```python
from build123d import *

# Parameters (mm, degrees)
PAD026_DEPTH      = 130
CYLINDER004_R     = 2.7
CYLINDER004_DEPTH = 30
CYLINDER005_R     = 2.7
CYLINDER005_DEPTH = 30
CYLINDER006_R     = 2.7
CYLINDER006_DEPTH = 30
CYLINDER007_R     = 2.7
CYLINDER007_DEPTH = 30
CYLINDER008_R     = 2.7
CYLINDER008_DEPTH = 30
CYLINDER009_R     = 2.7
CYLINDER009_DEPTH = 30
CYLINDER010_R     = 3.2
CYLINDER010_DEPTH = 50
CYLINDER011_R     = 3.2
CYLINDER011_DEPTH = 40
CYLINDER012_R     = 3.2
CYLINDER012_DEPTH = 40
CYLINDER013_R     = 7.5
CYLINDER013_DEPTH = 13
CYLINDER014_R     = 7.5
CYLINDER014_DEPTH = 13
CYLINDER015_R     = 7.5
CYLINDER015_DEPTH = 13
FILLET021_R       = 3


with BuildPart() as part:
    # Sketch051 → Pad026 (new body)
    with BuildSketch(Plane.XZ):
        Polygon((0, 0), (0, 20), (20, 20), (68.296291, 7.059048), (71.763809, 20), (110, 20), (110, 0), align=None)
    extrude(amount=PAD026_DEPTH)

    # Cylinder004 → Cylinder004 (cut)
    with BuildSketch(Plane(origin=(9, -10, 0), x_dir=(1, 0, 0), z_dir=(0, 0, 1))):
        Circle(CYLINDER004_R)
    extrude(amount=CYLINDER004_DEPTH, mode=Mode.SUBTRACT)

    # Cylinder005 → Cylinder005 (cut)
    with BuildSketch(Plane(origin=(95, -20, 0), x_dir=(1, 0, 0), z_dir=(0, 0, 1))):
        Circle(CYLINDER005_R)
    extrude(amount=CYLINDER005_DEPTH, mode=Mode.SUBTRACT)

    # Cylinder006 → Cylinder006 (cut)
    with BuildSketch(Plane(origin=(95, -65, 0), x_dir=(1, 0, 0), z_dir=(0, 0, 1))):
        Circle(CYLINDER006_R)
    extrude(amount=CYLINDER006_DEPTH, mode=Mode.SUBTRACT)

    # Cylinder007 → Cylinder007 (cut)
    with BuildSketch(Plane(origin=(95, -110, 0), x_dir=(1, 0, 0), z_dir=(0, 0, 1))):
        Circle(CYLINDER007_R)
    extrude(amount=CYLINDER007_DEPTH, mode=Mode.SUBTRACT)

    # Cylinder008 → Cylinder008 (cut)
    with BuildSketch(Plane(origin=(9, -65, 0), x_dir=(1, 0, 0), z_dir=(0, 0, 1))):
        Circle(CYLINDER008_R)
    extrude(amount=CYLINDER008_DEPTH, mode=Mode.SUBTRACT)

    # Cylinder009 → Cylinder009 (cut)
    with BuildSketch(Plane(origin=(9, -120, 0), x_dir=(1, 0, 0), z_dir=(0, 0, 1))):
        Circle(CYLINDER009_R)
    extrude(amount=CYLINDER009_DEPTH, mode=Mode.SUBTRACT)

    # Cylinder010 → Cylinder010 (cut)
    with BuildSketch(Plane(origin=(38, -35, -5), x_dir=(0.965926, 0, -0.258819), z_dir=(0.258819, 0, 0.965926))):
        Circle(CYLINDER010_R)
    extrude(amount=CYLINDER010_DEPTH, mode=Mode.SUBTRACT)

    # Cylinder011 → Cylinder011 (cut)
    with BuildSketch(Plane(origin=(38, -65, -5), x_dir=(0.965926, 0, -0.258819), z_dir=(0.258819, 0, 0.965926))):
        Circle(CYLINDER011_R)
    extrude(amount=CYLINDER011_DEPTH, mode=Mode.SUBTRACT)

    # Cylinder012 → Cylinder012 (cut)
    with BuildSketch(Plane(origin=(38, -100, -5), x_dir=(0.965926, 0, -0.258819), z_dir=(0.258819, 0, 0.965926))):
        Circle(CYLINDER012_R)
    extrude(amount=CYLINDER012_DEPTH, mode=Mode.SUBTRACT)

    # Cylinder013 → Cylinder013 (cut)
    with BuildSketch(Plane(origin=(38, -35, -5), x_dir=(0.965926, 0, -0.258819), z_dir=(0.258819, 0, 0.965926))):
        Circle(CYLINDER013_R)
    extrude(amount=CYLINDER013_DEPTH, mode=Mode.SUBTRACT)

    # Cylinder014 → Cylinder014 (cut)
    with BuildSketch(Plane(origin=(38, -65, -5), x_dir=(0.965926, 0, -0.258819), z_dir=(0.258819, 0, 0.965926))):
        Circle(CYLINDER014_R)
    extrude(amount=CYLINDER014_DEPTH, mode=Mode.SUBTRACT)

    # Cylinder015 → Cylinder015 (cut)
    with BuildSketch(Plane(origin=(38, -100, -5), x_dir=(0.965926, 0, -0.258819), z_dir=(0.258819, 0, 0.965926))):
        Circle(CYLINDER015_R)
    extrude(amount=CYLINDER015_DEPTH, mode=Mode.SUBTRACT)

    # Fillet021
    fillet021_edges = [part.edges().sort_by_distance(p)[0] for p in [
        (0, -65, 20),
        (110, -65, 20),
        (0, -130, 10),
        (110, -130, 10),
        (0, 0, 10),
        (110, 0, 10),
        (90.881905, -130, 20),
        (90.881905, 0, 20),
        (10, -130, 20),
        (10, 0, 20),
    ]]
    fillet(fillet021_edges, radius=FILLET021_R)


solid = part.part
```
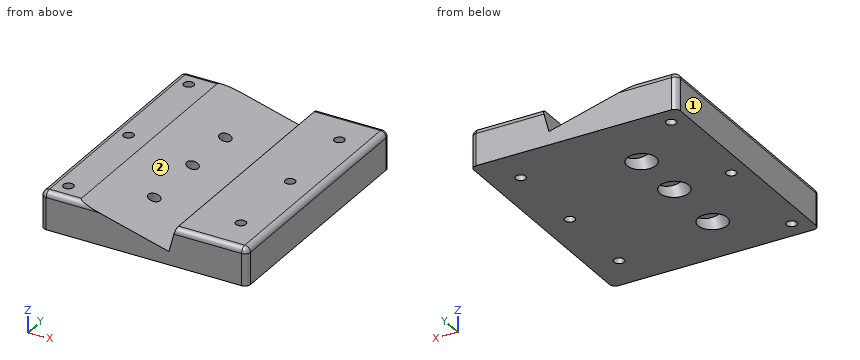
Part model, mm, in its own coordinate system. Face numbers are marked on the shaded views. A direction names the side the tool comes from. Coordinates: 2 decimals unless noted, no trailing zeros. Write each loop counter-clockwise with the first axis right and the second up, starting at its lowest first coordinate (ties: lowest second). Pieces come first, ordered by that corner, then holes.
Item 1: Which spindle directions (+Z, -Z, +X, -X, +Y, -Y) get a long thin tool onto all of the face, cutting with end or side? Do the marked faces 1 and 2. Say none if no direction does.
Item 2: Slice it at C-C (y = -65). Write the cut outline in (x, z).
Item 3: Slice it at D-D (y = -50). Write the cut outline in (x, z).
Item 4: Pin check, flat tip, straight feed: pin 1 (10 mm diameter, centred on x = 45, y = -32.5, fed in from +Z). Stop position of the tip, or through.
Item 5: Slice it at B-B (x = 95). Write the cut outline in (y, z), and give its area (3 significant figures).
Item 6: Slice it at A-A (y = -10). Write the cut outline in (x, z), and give its area (3 significant figures).
Item 7: Probe line 1 (Y direction, x = 9, z = 12); line 2 (Y direction, x = 95, z = 11.5); line 3 (X direction, y = -110, z = 6). List the from-to ranges inside material, lowest first.
Results found:
1. face 1: +Z, -Z, -X, +Y, -Y
1. face 2: +Z, +Y, -Y
2. outline: (0, 0) - (6.3, 0) - (6.3, 20) - (3, 20) arc R3 ccw to (0, 17) - close; (11.7, 0) - (31.58, 0) - (34.12, 9.5) - (38.27, 8.39) - (39.95, 14.65) - (20, 20) - (11.7, 20) - close; (44.46, 6.73) - (48.61, 5.62) - (47.1, 0) - (92.3, 0) - (92.3, 20) - (71.76, 20) - (68.3, 7.06) - (46.14, 13) - close; (97.7, 0) - (110, 0) - (110, 17) arc R3 ccw to (107, 20) - (97.7, 20) - close
3. outline: (0, 0) - (110, 0) - (110, 17) arc R3 ccw to (107, 20) - (71.76, 20) - (68.3, 7.06) - (20, 20) - (3, 20) arc R3 ccw to (0, 17) - close
4. pin 1: stops at z = 14.64
5. outline: (-130, 0) - (-112.7, 0) - (-112.7, 20) - (-127, 20) arc R3 ccw to (-130, 17) - close; (-107.3, 0) - (-67.7, 0) - (-67.7, 20) - (-107.3, 20) - close; (-62.3, 0) - (-22.7, 0) - (-22.7, 20) - (-62.3, 20) - close; (-17.3, 0) - (0, 0) - (0, 17) arc R3 ccw to (-3, 20) - (-17.3, 20) - close
5. area: 2,270 mm2
6. outline: (0, 0) - (6.3, 0) - (6.3, 20) - (3, 20) arc R3 ccw to (0, 17) - close; (11.7, 0) - (110, 0) - (110, 17) arc R3 ccw to (107, 20) - (71.76, 20) - (68.3, 7.06) - (20, 20) - (11.7, 20) - close
6. area: 1,750 mm2
7. line 1: y = -130 to -122.7, -117.3 to -67.7, -62.3 to -12.7, -7.3 to 0
7. line 2: y = -130 to -112.7, -107.3 to -67.7, -62.3 to -22.7, -17.3 to 0
7. line 3: x = 0 to 92.3, 97.7 to 110
